Can you work these out from the model? Positions are in its coordinate system, mm. A direction names the side the tool comes from. Coordinates: 2 decimals unless noted, no trailing zeros. Order: outer loops, then holes, each group sorted by start corner. A loop starts at its lowest first (then second) coordinate and runs counter-clockwise, first axis right, second up.
Autodesk Fusion 360 part; units mm, degrees
sketch "Sketch1" plane through (0, 0, 0) normal (0, 0, 1) x (1, 0, 0)
  line L0 (36, 35) -> (-36, 35)
  line L1 (-36, 35) -> (-36, -35)
  line L2 (-36, -35) -> (36, -35)
  line L3 (36, -35) -> (36, 35)
  line L4 (36, 35) -> (-36, -35) construction
  line L5 (-36, 35) -> (36, -35) construction
  dimension "d1" = 72
  dimension "d2" = 70
extrude "Extrude1" add sketch "Sketch1" along normal blind 30
shell "Shell1" thickness 2 removed faces 1 at (-12, 11.6667, 30)
sketch "Sketch2" plane through (-36, 0, 0) normal (-1, 0, 0) x (0, -1, 0)
  line L0 (-35, 0) -> (35, 0)
  line L1 (35, 0) -> (35, 30)
  line L2 (35, 30) -> (-35, 30)
  line L3 (-35, 30) -> (-35, 0)
  line L4 (35, 0) -> (17, 0)
  line L5 (17, 0) -> (17, 10)
  dimension "d11" = 18
  dimension "d12" = 10
hole "Hole2" at (-36, -17.0122, 10.0373) direction (1, 0, 0) diameter 5 depth 2 tip angle 118
sketch "Sketch3" plane through (0, -35, 0) normal (0, -1, 0) x (1, 0, 0)
  line L0 (-36, 0) -> (36, 0)
  line L1 (36, 0) -> (36, 30)
  line L2 (36, 30) -> (-36, 30)
  line L3 (-36, 30) -> (-36, 0)
hole "Hole3" at (6, -35, 15) direction (0, 1, 0) diameter 10 depth 2 tip angle 118
1. On a 3-axis mill with a long thin cutter (end or side, diameter ignored), from which of +Z, -Z, +X, -X, +Y, -Y can I reach the whole of each face in a straight line? I mean faces 1 (the flat face through (-36, 0, 15)), 2 (the flat face through (-34, 0, 16)), 3 (the cylindrical face through (6, -34, 20)). Say none if no direction works.
Completed:
face 1: +Z, -Z, -X, +Y, -Y
face 2: +Z
face 3: -Y
2. Imagine slicing it at C-C on y = 2. Please give me the cut outline in (x, z), then the cut area to 3 significant figures.
Completed:
outline: (-36, 0) - (36, 0) - (36, 30) - (34, 30) - (34, 2) - (-34, 2) - (-34, 30) - (-36, 30) - close
area: 256 mm2
3. Imagine slicing it at B-B on z = 21.5. Please give me the cut outline in (x, y), then the cut area to 3 significant figures.
Completed:
outline: (-36, -35) - (36, -35) - (36, 35) - (-36, 35) - close; hole (-34, -33) - (34, -33) - (34, 33) - (-34, 33) - close
area: 552 mm2
4. Thinking about a two-plate mould opening in Y: for faces 4 (the flat face through (-1, -35, 15)), 5 (the cylindrical face through (-34.99, -19.12, 11.38)), 6 (the flat face through (36, 0, 15)), which applies, pulls with the +Y half, pulls with the -Y half, needs draft (parallel to the pull), parting line crosses it, or undercut?
Completed:
face 4: pulls with the -Y half
face 5: undercut
face 6: needs draft
5. Imagine slicing it at D-D on z = 15. Please give me the cut outline in (x, y).
Completed:
outline: (-36, -35) - (1, -35) - (1, -33) - (-34, -33) - (-34, 33) - (34, 33) - (34, -33) - (11, -33) - (11, -35) - (36, -35) - (36, 35) - (-36, 35) - close
6. I'm going to push a flat-ended pin straight in: pin 1 (8 mm diameter, centred on x = -23, y = -5.5, fed in from +Z). Where does the tip first touch, or does it pass through?
Completed:
pin 1: stops at z = 2
7. Imagine slicing it at A-A on x = 6. Please give me the cut outline in (y, z), then the cut area to 3 significant figures.
Completed:
outline: (-35, 0) - (35, 0) - (35, 30) - (33, 30) - (33, 2) - (-33, 2) - (-33, 10) - (-35, 10) - close; (-35, 20) - (-33, 20) - (-33, 30) - (-35, 30) - close
area: 232 mm2
8. Please list where these lines run through material, in increasing order: probe 1 along X at (y, z) = (21, 5.5); probe 2 along Y at (x, z) = (-27, 20.75); probe 3 along Z at (x, y) = (6, -33.85).
Completed:
probe 1: x = -36 to -34, 34 to 36
probe 2: y = -35 to -33, 33 to 35
probe 3: z = 0 to 10, 20 to 30
